```python
from build123d import *

# Parameters (mm, degrees)
SKETCH6_R          = 6.864817117
CUT_EXTRUDE2_DEPTH = 3.3
SKETCH5_R          = 50.459472618
CUT_EXTRUDE1_DEPTH = 25


# Read off the part's stored shape, not the designer's step: Split1
with BuildPart() as part:
    # Sketch1 → Revolve2 (revolve)
    with BuildSketch(Plane(origin=(0, 0, 0), x_dir=(0, 0, -1), z_dir=(1, 0, 0)), mode=Mode.PRIVATE) as revolve2_sk:
        with BuildLine():
            Line((1.771e-06, 9.5), (1.771e-06, 7.445611339))
            Line((1.771e-06, 7.445611339), (-0.771464581, 7.445611339))
            Line((-0.771464581, 7.445611339), (-0.771464581, 6.864817117))
            Line((-0.771464581, 6.864817117), (-4.066354879, 6.864817117))
            Line((-4.066354879, 6.864817117), (-4.066354879, 8.484339467))
            Line((-4.066354879, 8.484339467), (-4.975618005, 9.546154997))
            Line((-4.975618005, 9.546154997), (-7.06424338, 9.546154997))
            Line((-7.06424338, 9.546154997), (-7.767897919, 10.954193429))
            Line((-7.767897919, 10.954193429), (-9.164037876, 10.954193429))
            Line((-9.164037876, 10.954193429), (-9.945876251, 9.546154997))
            Line((-9.945876251, 9.546154997), (-9.945876251, 8))
            Line((-9.945876251, 8), (-19.896053439, 8))
            Line((-19.896053439, 8), (-20.566354879, 7.426001631))
            Line((-20.566354879, 7.426001631), (-23.121440557, 7.426001631))
            Line((-23.121440557, 7.426001631), (-23.682625072, 6.864817117))
            Line((-23.682625072, 6.864817117), (-23.682625072, 6.383537324))
            Line((-23.682625072, 6.383537324), (-27.0133813, 6.383537324))
            Line((-27.0133813, 6.383537324), (-27.0133813, 5.464238658))
            Line((-27.0133813, 5.464238658), (-31.931960755, 5.464238658))
            Line((-31.931960755, 5.464238658), (-31.931960755, 1.447456583))
            Line((-31.931960755, 1.447456583), (-38.111348046, 1.447456583))
            Line((-38.111348046, 1.447456583), (-38.931960755, 1.037362766))
            Line((-38.931960755, 1.037362766), (-38.931960755, 0))
            Line((-38.931960755, 0), (2.933645121, 0))
            ThreePointArc((2.933645121, 0), (2.489100327, 4.831124101), (1.170397182, 9.5))
            Line((1.170397182, 9.5), (1.771e-06, 9.5))
        make_face()
    revolve(revolve2_sk.sketch.rotate(Axis((0, 0, 38.931960755), (0, 0, -1)), 90), axis=Axis((0, 0, 38.931960755), (0, 0, -1)))


with BuildPart() as body_2:
    # Split1: the piece on the far side of the plane
    add(part.part)
    split(bisect_by=Plane.XY.offset(4.066354879), keep=Keep.BOTTOM)

    # Sketch5 → Cut-Extrude1 (cut)
    with BuildSketch(Plane(origin=(0, 0, 4.066354879), x_dir=(-1, 0, 0), z_dir=(0, 0, -1))):
        Circle(SKETCH5_R)
    extrude(amount=CUT_EXTRUDE1_DEPTH, mode=Mode.SUBTRACT)


with BuildPart() as part_1:
    add(part.part)

    # Split1
    split(bisect_by=Plane.XY.offset(4.066354879), keep=Keep.TOP)

    # Sketch6 → Cut-Extrude2 (cut)
    with BuildSketch(Plane(origin=(0, 0, 4.066354879), x_dir=(-1, 0, 0), z_dir=(0, 0, -1))):
        Circle(SKETCH6_R)
    extrude(amount=-CUT_EXTRUDE2_DEPTH, mode=Mode.SUBTRACT)


solid = part_1.part
```
For this review, take the finished solid that the model builds, in its own axes (mm). A direction names the side the tool comes from. Round coordinates to 2 decimals unless told otherwise and drop trailing zeros. Loops run counter-clockwise (first coordinate to the right, second up) from the corner with the lowest first, then second, coordinate; pieces in that order, holes last.
(1) Tool access review of faces 4 (the flat face through (0, 0, 7.366)), 5 (the flat face through (1, 7, 4.066)), 6 (the flat face through (1.14, 1.14, 31.932)): name each direction out of +Z, -Z, +X, -X, +Y, -Y from which nothing blocks a thin tool from reaching the whole face with its end or side.
Returned:
face 4: -Z
face 5: -Z, +X, -X, +Y, -Y
face 6: +Z
(2) Mouldability with a two-part tool opening along Y and no side actions: class faces 1 (the cylindrical face through (1.5, -6.7, 5.7)), 2 (the flat face through (-6, 6, 9.946)), 3 (the cylindrical face through (7.083, -2.231, 21.862)) as released by +Y, released by -Y, zero draft, split by the parting line, or undercut.
Returned:
face 1: undercut
face 2: zero draft
face 3: split by the parting line
(3) We need section A-A (z = 36.5). Give the boundary of the cut face in (x, y).
Returned:
outline: circle Ø2.89 at (0, 0)
(4) Clearance check with flat-ended pins moving along their axes: P1, Ø1.5, axis at y = 3.5, z = 35.5, coming from the +X side; P2, Ø3, axis at x = -3, y = -0.5, coming from the +Z side; P3, Ø5, axis at y = -5.5, z = 12.5, coming from the -X side; P4, Ø4, axis at x = -7.5, y = -5.5, coming from the +Z side. State where each tip first meets the part, or that it passes through.
Returned:
P1: passes through
P2: stops at z = 31.93
P3: stops at x = -7.42
P4: stops at z = 23.25
(5) We need section B-B (z = 24.5). Give the boundary of the cut face in (x, y), plus the area to 3 significant figures.
Returned:
outline: circle Ø12.77 at (0, 0)
area: 128 mm2
(6) Wall thickness on line 1 along Y through (x, z) = (0, 5.45); line 2 along Z through (x, y) = (2.5, -5); line 3 along Z through (x, y) = (4, 3.25): over which ranges is each line inside the solid? List them lowest first.
Returned:
line 1: y = -9.55 to -6.86, 6.86 to 9.55
line 2: z = 7.37 to 27.01
line 3: z = 7.37 to 31.93
